Check sheet for the modelled part. Datum: model origin and axes. Units: mm. Face numbers are marked on the shaded views. Round coordinates to 2 decimals unless told otherwise and drop trailing zeros. Write each loop counter-clockwise with the first axis right and the second up, starting at its lowest first coordinate (ties: lowest second). Pieces come first, ordered by that corner, then holes. Notation, with made-up numbers: (80.25, 68.5) -> (119.25, 68.5) arc R16 ccw to (119.25, 88.5) -> close; hole circle Ø1 at (27.5, 74). An arc over 180 degrees is marked (long way). One line per item, written item: value. Start each with the question number.
```python
from build123d import *

# Parameters (mm, degrees)
SCHIZZO1_W                   = 45
SCHIZZO1_H                   = 10
ESTRUSIONE_ESTRUSIONE1_DEPTH = 5
SCHIZZO2_R                   = 2.5
TAGLIO_ESTRUSIONE1_DEPTH     = 26.124689053


with BuildPart() as part:
    # Schizzo1 → Estrusione-Estrusione1 (new, symmetric)
    with BuildSketch(Plane.XY):
        with Locations((0, -36.584144653)):
            Rectangle(SCHIZZO1_W, SCHIZZO1_H)
    extrude(amount=ESTRUSIONE_ESTRUSIONE1_DEPTH, both=True)

    # Schizzo2 → Taglio-Estrusione1 (cut, through all)
    with BuildSketch(Plane.XZ.offset(41.584144653)):
        with Locations(Location((0.501094215, 0, 0), (0, 0, 270))):
            Circle(SCHIZZO2_R)
    extrude(amount=-TAGLIO_ESTRUSIONE1_DEPTH, mode=Mode.SUBTRACT)


solid = part.part
```
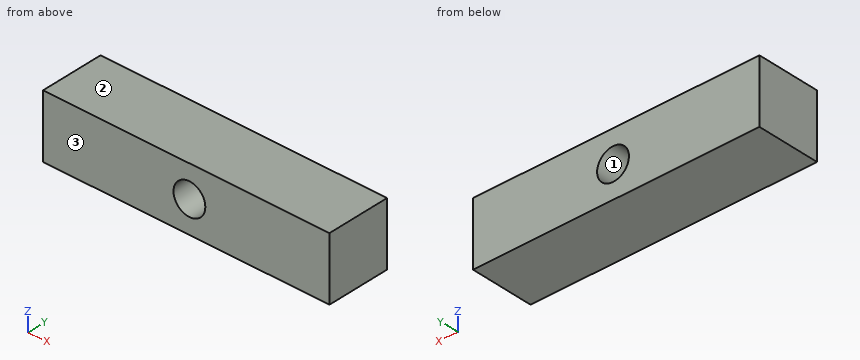
1. Material ranges on probe 1 along X at (y, z) = (-33, 0); probe 2 along X at (y, z) = (-32.5, -2); probe 3 along Z at (x, y) = (-1, -33.75), recorded low to high.
2. Release check for a two-part mould opening along Z. For the marked faces 1, 2 and 3 record: +Z half, -Z half, draft (parallel to the pull), parting line (faces both ways), or undercut.
3. Cross-section at A-A (z = 0). Record the cut outline in (x, y), plus the area to 3 significant figures.
4. Cross-section at B-B (y = -40.25). Record the cut outline in (x, z).
5. Cross-section at C-C (z = 1.75). Record the cut outline in (x, y).
Working result:
1. probe 1: x = -22.5 to -2, 3 to 22.5
1. probe 2: x = -22.5 to -1, 2 to 22.5
1. probe 3: z = -5 to -2, 2 to 5
2. face 1: undercut
2. face 2: +Z half
2. face 3: draft
3. outline: (-22.5, -41.58) -> (-2, -41.58) -> (-2, -31.58) -> (-22.5, -31.58) -> close; (3, -41.58) -> (22.5, -41.58) -> (22.5, -31.58) -> (3, -31.58) -> close
3. area: 400 mm^2
4. outline: (-22.5, -5) -> (22.5, -5) -> (22.5, 5) -> (-22.5, 5) -> close; hole circle Ø5 at (0.5, 0)
5. outline: (-22.5, -41.58) -> (-1.28, -41.58) -> (-1.28, -31.58) -> (-22.5, -31.58) -> close; (2.29, -41.58) -> (22.5, -41.58) -> (22.5, -31.58) -> (2.29, -31.58) -> close
